Here's how the part is built. I have some questions about the finished solid (model axes, mm). A direction names the side the tool comes from. Round coordinates to 2 decimals unless told otherwise and drop trailing zeros. Order: outer loops, then holes, each group sorted by start corner. A loop starts at its lowest first (then second) coordinate and runs counter-clockwise, first axis right, second up. Notation, with made-up numbers: (-27, 46) -> (14, 46) arc R26 cw to (14, 69) -> close; hole circle Ø3 at (-5.75, -3). An arc over 180 degrees is marked (long way). Answer in a Markdown table with one row per item.
Autodesk Inventor part; units mm, degrees
ref_plane "YZ Plane" through (0, 0, 0) normal (1, 0, 0) x (0, 1, 0)
ref_plane "XZ Plane" through (0, 0, 0) normal (0, 1, 0) x (-1, 0, 0)
ref_plane "XY Plane" through (0, 0, 0) normal (0, 0, 1) x (1, 0, 0)
sketch "Sketch1" plane through (0, 0, 0) normal (0, 0, 1) x (1, 0, 0)
  line L0 (-21.25, 21.25) -> (21.25, 21.25)
  line L1 (21.25, 21.25) -> (21.25, -21.25)
  line L2 (21.25, -21.25) -> (-21.25, -21.25)
  line L3 (-21.25, -21.25) -> (-21.25, 21.25)
  line L4 (-21.25, 21.25) -> (21.25, -21.25) construction
  line L5 (21.25, 21.25) -> (-21.25, -21.25) construction
  circle A0 centre (0, 0) radius 11 construction
  circle A1 centre (0, 0) radius 12.5
  line L6 (-25.25, 3.5236) -> (25.25, 3.5236)
  line L7 (25.25, 3.5236) -> (25.25, 25.25)
  line L8 (25.25, 25.25) -> (-25.25, 25.25)
  line L9 (-25.25, 25.25) -> (-25.25, 3.5236)
  circle A2 centre (-15.5, 15.5) radius 1.5
  circle A3 centre (15.5, 15.5) radius 1.5
  point P0 (21.25, 3.5236)
  point P1 (-21.25, 3.5236)
  dimension "d0" = 42.5
  dimension "d1" = 42.5
  dimension "d2" = 22
  dimension "d3" = 25
  dimension "d4" = 4
  dimension "d5" = 4
  dimension "d6" = 4
  dimension "d7" = 3
  dimension "d8" = 3
  dimension "d9" = 15.5
  dimension "d10" = 15.5
  dimension "d11" = 15.5
  dimension "d12" = 15.5
extrude "Extrusion1" add sketch "Sketch1" along normal blind 4 contours L3 L6 L9 L8 L7 L1 L0 | L0 L1 L6 A1 L3 | A1 L6 picked at (3.04, 5.1985)
extrude "Extrusion2" cut sketch "Sketch1" along normal blind 4 contours L6 A1 | A1 L6
extrude "Extrusion3" add sketch "Sketch1" against normal blind 8 contours L3 L6 L9 L8 L7 L1 L0
sketch "Sketch2" plane through (0, 0, 4) normal (0, 0, 1) x (1, 0, 0)
  circle A0 centre (0, 0) radius 40 construction
  line L0 (-25.25, 3.5236) -> (25.25, 3.5236) construction
  line L1 (-25.25, 3.5236) -> (-11.9931, 3.5236)
  line L2 (-25.25, 3.5236) -> (25.25, 3.5236)
  line L3 (39.8445, 92.8978) -> (39.8445, 152.8119)
  line L4 (39.8445, 152.8119) -> (-39.8445, 152.8119)
  line L5 (-39.8445, 152.8119) -> (-39.8445, 92.8978)
  circle A1 centre (-15.5, 15.5) radius 1.5
  circle A2 centre (-15.5, 15.5) radius 1.5
  circle A3 centre (15.5, 15.5) radius 1.5
  circle A4 centre (15.5, 15.5) radius 1.5
  line L6 (25.25, 54.4811) -> (25.25, 3.5236)
  line L7 (25.25, 54.4811) -> (25.25, -31.0232) construction
  line L8 (-25.25, 25.25) -> (-25.25, -31.0232) construction
  line L9 (25.25, 3.5236) -> (25.25, 54.4811)
  line L10 (25.25, 3.5236) -> (25.25, 54.4811) construction
  line L11 (25.25, 54.4811) -> (39.8445, 54.4811) construction
  line L12 (39.8445, 54.4811) -> (39.8445, 92.8978) construction
  spline S0 degree 3 poles (25.25, 3.5236) (25.25, 54.4811) (39.8445, 54.4811) (39.8445, 92.8978) knots 1 1 1 1 2 2 2 2
  line L13 (-25.25, 3.5236) -> (-25.25, 54.4811) construction
  line L14 (-25.25, 54.4811) -> (-39.8445, 54.4811) construction
  line L15 (-39.8445, 54.4811) -> (-39.8445, 92.8978) construction
  spline S1 degree 3 poles (-25.25, 3.5236) (-25.25, 54.4811) (-39.8445, 54.4811) (-39.8445, 92.8978) knots 1 1 1 1 2 2 2 2
  point P0 (-39.8445, 3.5236)
  point P1 (39.8445, 3.5236)
  dimension "d19" = 80
  dimension "d20" = 150
  dimension "d21" = 39.8445
extrude "Extrusion4" add sketch "Sketch2" against normal blind 4
fillet "Fillet1" radius 20 2 edges at (-39.8445, 152.8119, 2) (39.8445, 152.8119, 2)
equation "\"d1\" = d0"
equation "\"d5\" = d4"
equation "\"d6\" = d4"
equation "\"d8\" = d7"
equation "\"d11\" = d9"
properties part number "Sideplate"
1. For faces 1 (the face through (0, 25.25, -4)), 2 (the face through (39.844, 113, 2)), 3 (the face through (14, 15.43, 1.97)), 4 (the face through (0, 21.25, -4)), 5 (the face through (-25.25, 15, -4)), which set-ups out of +Z, -Z, +X, -X, +Y, -Y let a thin tool reach every point of the face, with its end or its side?
Numbers:
| item | result |
|---|---|
| face 1 | -Z, +X, -X, +Y |
| face 2 | +Z, -Z, +X, +Y, -Y |
| face 3 | +Z, -Z |
| face 4 | -Z, -Y |
| face 5 | -Z, -X, +Y, -Y |
2. For pin 1 Ø4 at (x, z) = (-5.5, -2.5) entering from -Y; pin 2 Ø6 at (x, y) = (-13, 119) entering from -Z; pin 3 Ø6.5 at (x, z) = (-7.5, -4) entering from +Y, each with a flat end and sliding along its axis, tell me the tip position at first contact or that it passes through.
Numbers:
| item | result |
|---|---|
| pin 1 | stops at y = 21.25 |
| pin 2 | stops at z = 0 |
| pin 3 | stops at y = 25.25 |
3. We'd pull the mould along X, two halves only. Please class faces 6 (the face through (-21.25, 12, -4)), 7 (the face through (0, 3.524, 1)), 8 (the face through (25.25, 14, -4)): released by +X, released by -X, zero draft, split by the parting line, or undercut.
Numbers:
| item | result |
|---|---|
| face 6 | undercut |
| face 7 | zero draft |
| face 8 | released by +X |
4. Suppose I cut it at B-B on z = -5.5. Write out the boundary of the cut face in (x, y).
Numbers:
| item | result |
|---|---|
| outline | (-25.25, 3.52) -> (-21.25, 3.52) -> (-21.25, 21.25) -> (21.25, 21.25) -> (21.25, 3.52) -> (25.25, 3.52) -> (25.25, 25.25) -> (-25.25, 25.25) -> close |
5. Suppose I cut it at C-C on y = 104. Write out the boundary of the cut face in (x, z).
Numbers:
| item | result |
|---|---|
| outline | (-39.84, 0) -> (39.84, 0) -> (39.84, 4) -> (-39.84, 4) -> close |
6. Please list where these lines run through material, in increasing order: line 1 along Y through (x, z) = (-15.5, 1.2); line 2 along Z through (x, y) = (-13.5, 110); line 3 along Y through (x, z) = (4, -3.5).
Numbers:
| item | result |
|---|---|
| line 1 | y = 3.52 to 14, 17 to 152.81 |
| line 2 | z = 0 to 4 |
| line 3 | y = 21.25 to 25.25 |
7. Suppose I cut it at D-D on z = 2. State how many separate pieces and enclosed holes the cut face has, then the cut area to 3 significant figures.
Numbers:
| item | result |
|---|---|
| separate pieces | 1 |
| enclosed holes | 2 |
| area | 10,300 mm2 |
8. Suppose I cut it at A-A on x = 15.5. Write out the boundary of the cut face in (y, z).
Numbers:
| item | result |
|---|---|
| outline | (3.52, 0) -> (14, 0) -> (14, 4) -> (3.52, 4) -> close; (17, 0) -> (21.25, 0) -> (21.25, -8) -> (25.25, -8) -> (25.25, 0) -> (152.81, 0) -> (152.81, 4) -> (17, 4) -> close |
